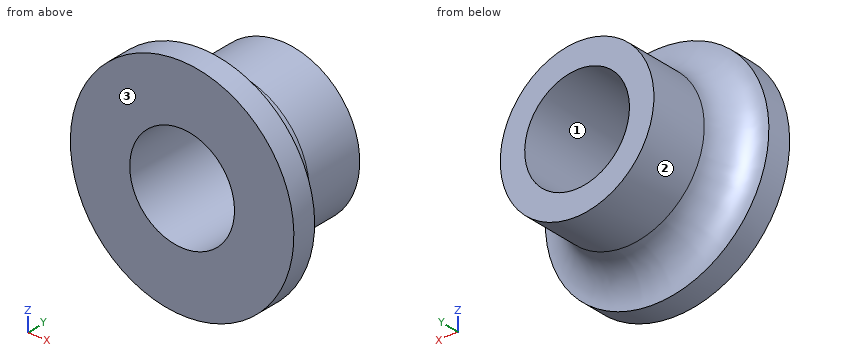
from build123d import *

# Parameters (mm, degrees)
SKETCH_1_R      = 16
SKETCH_1_R_2    = 7.5
EXTRUDE_1_DEPTH = 3.5
SKETCH_2_R      = 11
SKETCH_2_R_2    = 7.5
EXTRUDE_2_DEPTH = 13.5
FILLET_1_R      = 5


with BuildPart() as part:
    # 草圖1 → 填料-伸長1 (new body)
    with BuildSketch(Plane(origin=(0, 0, 0), x_dir=(1, 0, 0), z_dir=(0, 1, 0))):
        with Locations(Location((0, 0, 0), (0, 0, 270))):
            Circle(SKETCH_1_R)
        with Locations(Location((0, 0, 0), (0, 0, 270))):
            Circle(SKETCH_1_R_2, mode=Mode.SUBTRACT)
    extrude(amount=EXTRUDE_1_DEPTH)

    # 草圖2 → 填料-伸長2 (add)
    with BuildSketch(Plane(origin=(0, 3.5, 0), x_dir=(1, 0, 0), z_dir=(0, 1, 0))):
        with Locations(Location((0, 0, 0), (0, 0, 270))):
            Circle(SKETCH_2_R)
        with Locations(Location((0, 0, 0), (0, 0, 270))):
            Circle(SKETCH_2_R_2, mode=Mode.SUBTRACT)
    extrude(amount=EXTRUDE_2_DEPTH)

    # 圓角1
    fillet_1_edges = [part.edges().sort_by_distance(p)[0] for p in [
        (0, 3.5, -11),
    ]]
    fillet(fillet_1_edges, radius=FILLET_1_R - 0.0001)  # a hair under: the kernel refuses the full size


solid = part.part
Read the model definition and answer for the solid it produces. Units are mm, in the model's axes. Face numbers are marked on the shaded views. Coordinates: 2 decimals unless noted, no trailing zeros. Order: outer loops, then holes, each group sorted by start corner. A loop starts at its lowest first (then second) coordinate and runs counter-clockwise, first axis right, second up. Notation, with made-up numbers: (1, -38.75) -> (21, -38.75) arc R4 ccw to (21, -34.75) -> close; hole circle Ø5 at (-29.5, 9.25). An arc over 180 degrees is marked (long way). Answer as a JSON object with one key per item and string values.
1) A cutting plane is placed at D-D, the plane y = 12.75. Determine the outline of the cut face in (x, z), plus the area to 3 significant figures.
Model answer:
{"outline": "circle Ø22 at (0, 0); hole circle Ø15 at (0, 0)", "area": "203 mm²"}
2) Each of these flat-tipped pins is pushed along its axis until it touches: pin 1 (10 mm diameter, centred on x = 0, y = 8, fed in from +Z); pin 2 (10 mm diameter, centred on x = 9.5, y = 14, fed in from -Z). Where does it stop, or does it pass through?
Model answer:
{"pin 1": "stops at z = 16", "pin 2": "stops at z = -10.04"}
3) The mould has two halves that part along X. Classify the marked faces 1, 2 and 3: released by +X, released by -X, zero draft, split by the parting line, or undercut.
Model answer:
{"face 1": "undercut", "face 2": "split by the parting line", "face 3": "zero draft"}
4) A cutting plane is placed at C-C, the plane y = 3. Determine the outline of the cut face in (x, z), plus the area to 3 significant figures.
Model answer:
{"outline": "circle Ø32 at (0, 0); hole circle Ø15 at (0, 0)", "area": "628 mm²"}
5) Consider line 1 along X through (y, z) = (8.25, 0); line 2 along X through (y, z) = (7.75, 0); line 3 along Z through (x, y) = (-3.5, 15.5). Determine where each line is inside the solid, lowest interval first. Write a range as from..to.
Model answer:
{"line 1": "x = -11.01..-7.5, 7.5..11.01", "line 2": "x = -11.06..-7.5, 7.5..11.06", "line 3": "z = -10.43..-6.63, 6.63..10.43"}
